Geometry check sheet. Reference: the model listing, model coordinates, mm. A direction names the side the tool comes from. Coordinates: 2 decimals unless noted, no trailing zeros. Write each loop counter-clockwise with the first axis right and the second up, starting at its lowest first coordinate (ties: lowest second). Pieces come first, ordered by that corner, then holes. Notation, with made-up numbers: M -25,-9.75 L 20,-9.75 A22 ccw 20,28.25 Z; hole C 59.5,5 d3. An arc over 180 degrees is marked long. Write item = value, one per line. Start each with the question number.
Autodesk Inventor part; units mm, degrees
ref_plane "YZ Plane" through (0, 0, 0) normal (1, 0, 0) x (0, 1, 0)
ref_plane "XZ Plane" through (0, 0, 0) normal (0, 1, 0) x (-1, 0, 0)
ref_plane "XY Plane" through (0, 0, 0) normal (0, 0, 1) x (1, 0, 0)
sketch "Sketch1" plane through (0, 0, 0) normal (1, 0, 0) x (0, 1, 0)
  line L0 (0, 0) -> (-33.7, 0)
  line L1 (0, 0) -> (0, -4.3)
  arc A0 (-1.5, -4.5) -> (-0.5, -4.5) centre (-1, -4.5) ccw
  line L2 (-0.5, -4.5) -> (-0.5, -4.3)
  line L3 (-1.5, -4.5) -> (-1.5, -4.3)
  line L4 (0, -4.3) -> (-0.5, -4.3)
  line L5 (-1.5, -4.3) -> (-2, -4.3)
  line L6 (-2, -4.3) -> (-2.5, -4.3)
  arc A1 (-3.5, -4.5) -> (-2.5, -4.5) centre (-3, -4.5) ccw
  line L7 (-2.5, -4.5) -> (-2.5, -4.3)
  line L8 (-3.5, -4.5) -> (-3.5, -4.3)
  line L9 (-3.5, -4.3) -> (-4, -4.3)
  line L10 (-4, -4.3) -> (-4.5, -4.3)
  arc A2 (-5.5, -4.5) -> (-4.5, -4.5) centre (-5, -4.5) ccw
  line L11 (-4.5, -4.5) -> (-4.5, -4.3)
  line L12 (-5.5, -4.5) -> (-5.5, -4.3)
  line L13 (-5.5, -4.3) -> (-6, -4.3)
  line L14 (-6, -4.3) -> (-6.5, -4.3)
  arc A3 (-7.5, -4.5) -> (-6.5, -4.5) centre (-7, -4.5) ccw
  line L15 (-6.5, -4.5) -> (-6.5, -4.3)
  line L16 (-7.5, -4.5) -> (-7.5, -4.3)
  line L17 (-7.5, -4.3) -> (-8, -4.3)
  line L18 (-8, -4.3) -> (-8.5, -4.3)
  arc A4 (-9.5, -4.5) -> (-8.5, -4.5) centre (-9, -4.5) ccw
  line L19 (-8.5, -4.5) -> (-8.5, -4.3)
  line L20 (-9.5, -4.5) -> (-9.5, -4.3)
  line L21 (-9.5, -4.3) -> (-10, -4.3)
  line L22 (-10, -4.3) -> (-10.5, -4.3)
  arc A5 (-11.5, -4.5) -> (-10.5, -4.5) centre (-11, -4.5) ccw
  line L23 (-10.5, -4.5) -> (-10.5, -4.3)
  line L24 (-11.5, -4.5) -> (-11.5, -4.3)
  line L25 (-11.5, -4.3) -> (-12, -4.3)
  line L26 (-12, -4.3) -> (-12.5, -4.3)
  arc A6 (-13.5, -4.5) -> (-12.5, -4.5) centre (-13, -4.5) ccw
  line L27 (-12.5, -4.5) -> (-12.5, -4.3)
  line L28 (-13.5, -4.5) -> (-13.5, -4.3)
  line L29 (-13.5, -4.3) -> (-14, -4.3)
  line L30 (-14, -4.3) -> (-14.5, -4.3)
  arc A7 (-15.5, -4.5) -> (-14.5, -4.5) centre (-15, -4.5) ccw
  line L31 (-14.5, -4.5) -> (-14.5, -4.3)
  line L32 (-15.5, -4.5) -> (-15.5, -4.3)
  line L33 (-15.5, -4.3) -> (-16, -4.3)
  line L34 (-16, -4.3) -> (-16.5, -4.3)
  arc A8 (-17.5, -4.5) -> (-16.5, -4.5) centre (-17, -4.5) ccw
  line L35 (-16.5, -4.5) -> (-16.5, -4.3)
  line L36 (-17.5, -4.5) -> (-17.5, -4.3)
  line L37 (-17.5, -4.3) -> (-18, -4.3)
  line L38 (-18, -4.3) -> (-18.5, -4.3)
  arc A9 (-19.5, -4.5) -> (-18.5, -4.5) centre (-19, -4.5) ccw
  line L39 (-18.5, -4.5) -> (-18.5, -4.3)
  line L40 (-19.5, -4.5) -> (-19.5, -4.3)
  line L41 (-19.5, -4.3) -> (-20, -4.3)
  line L42 (-20, -5.7) -> (0, -5.7)
  line L43 (0, -5.7) -> (0, -10)
  line L44 (0, -10) -> (-33.7, -10)
  line L45 (-33.7, -10) -> (-33.7, 0)
  line L46 (-20, -5) -> (0, -5) construction
  arc A10 (-24.3, 0) -> (-20, -4.3) centre (-20, 0) ccw
  arc A11 (-25.7, 0) -> (-20, -5.7) centre (-20, 0) ccw
  dimension "d1" = 2
  dimension "d2" = 1
  dimension "d4" = 1
  dimension "d5" = 0.2
  dimension "d8" = 2
  dimension "d14" = 1.4
  dimension "d15" = 10
  dimension "d31" = 8
extrude "Extrusion1" add sketch "Sketch1" along normal blind 10
sketch "Sketch2" plane through (0, -33.7, -10) normal (0, -1, 0) x (1, 0, 0)
  line L0 (0, 10) -> (0, 0) construction
  line L1 (0, 0) -> (10, 0) construction
  line L2 (10, 10) -> (10, 0) construction
  line L3 (0, 10) -> (10, 10) construction
  line L4 (0, 0) -> (10, 0) construction
  line L5 (0, 5.7) -> (0, 10) construction
  line L6 (10, 0) -> (0, 10) construction
  line L7 (0, 10) -> (10, 10) construction
  line L8 (10, 10) -> (0, 0) construction
  line L9 (0, 5) -> (10, 5) construction
  point P0 (5, 5)
hole "Hole1" at (5, -33.7, -5) direction (0, 1, 0) diameter 4.3 depth 8
sketch "Sketch3" plane through (0, 0, 0) normal (-1, 0, 0) x (0, 0, 1)
  line L0 (-10, -33.7) -> (-10, 0) construction
  line L1 (0, 0) -> (0, -33.7) construction
  line L2 (0, -33.7) -> (-10, -33.7)
  line L3 (-4.3, 0) -> (0, 0)
  line L4 (-10, -33.7) -> (0, -33.7)
  line L5 (0, -33.7) -> (0, 0)
  line L6 (0, 0) -> (-10, 0)
  line L7 (-10, 0) -> (-10, -33.7)
  line L8 (-10, -33.7) -> (-10, 0)
  line L9 (0, 0) -> (0, -33.7)
  arc A0 (-5.7, -20) -> (0, -25.7) centre (0, -20) ccw
  line L10 (0, -25.7) -> (-10, -25.7)
  point P0 (-4.3, 0)
  point P1 (0, -25.7)
extrude "Extrusion2" add sketch "Sketch3" against normal blind 4 contours L10 L7 L6 L3 L5
sketch "Sketch5" plane through (0, 0, 0) normal (-1, 0, 0) x (0, 0, 1)
  line L0 (-3.5, 0) -> (0, -13.0622)
  line L1 (-6.5, 0) -> (-10, -13.0622)
  line L2 (0, 0) -> (0, -33.7)
  line L3 (-10, 0) -> (0, 0)
  line L4 (-10, -33.7) -> (-10, 0)
  line L5 (0, -33.7) -> (-10, -33.7)
  line L6 (-5, 0) -> (-5, -33.7) construction
  line L7 (0, -33.7) -> (-10, -33.7)
  dimension "d33" = 3
  dimension "d34" = 15
properties part number "BeltClampTensioner"
Q1. Gauge pin test, flat ends, axial feed: pin 1 (4 mm diameter, centred on x = 5, z = -5, fed in from +Y); pin 2 (2 mm diameter, centred on x = 4.5, z = -5.5, fed in from -Y). Record the tip position at first contact, or that the pin passes through.
Q2. Scan lines: L1, parallel to X at y = -28, z = -5; L2, parallel to Z at x = 5, y = -29.5; L3, parallel to Z at x = 6.5, y = -23. Record each from-to range of solid material in increasing order.
Q3. Set-up check for faces 3 (the face through (7, -4, -4.3)), 4 (the face through (6.308, -29.644, -3.294)), 5 (the face through (7, -10, -5.7)), 6 (the face through (5, -17, -10)), 7 (the face through (10, -21, -6)): record each of +Z, -Z, +X, -X, +Y, -Y from which the full face is reachable in a straight line by a thin tool's end or side.
Q4. Cross-section at B-B on y = -27. Enter the section's corners in (x, z).
Q5. Cross-section at A-A on y = -8. Enter the section's corners in (x, z), and give its area (3 significant figures).
Q6. Draft check along Y on faces 1 (the face through (7, -17, -5)), 2 (the face through (5, -17, 0)). Enter one of: pulls with the +Y half, pulls with the -Y half, needs draft (parallel to the pull), parting line crosses it, or undercut.
Q7. Cross-section at C-C on y = -3. Enter the section's corners in (x, z), and give its area (3 significant figures).
Values found:
q1.pin_1 = 0
q1.pin_2 = -25.7
q2.L1 = 0 to 2.85, 7.15 to 10
q2.L2 = -10 to -7.15, -2.85 to 0
q2.L3 = -10 to -4.85, -3.08 to 0
q3.face_3 = +X
q3.face_4 = -Y
q3.face_5 = +X, +Y
q3.face_6 = -Z, +X, -X, +Y, -Y
q3.face_7 = +Z, -Z, +X, +Y, -Y
q4.outline = M 0,-10 L 10,-10 L 10,0 L 0,0 Z; hole C 5,-5 d4.3
q5.outline = M 0,-10 L 10,-10 L 10,-5.7 L 4,-5.7 L 4,-4.3 L 10,-4.3 L 10,0 L 0,0 Z
q5.area = 91.6 mm²
q6.face_1 = undercut
q6.face_2 = needs draft
q7.outline = M 0,-10 L 10,-10 L 10,-5.7 L 4,-5.7 L 4,-5 L 10,-5 L 10,0 L 0,0 Z
q7.area = 95.8 mm²
